Geometry: final body of the model. Coordinates: model frame, mm. A direction names the side the tool comes from. Give positions to 0.01 mm unless a question says otherwise; leave off trailing zeros. Write each loop counter-clockwise with the first axis right and the second up, starting at its lowest first coordinate (ties: lowest second). Pieces come first, ordered by that corner, then holes. Notation, with made-up numbers: (56, 55.25) -> (76, 55.25) arc R26 ccw to (76, 75.25) -> close; hole circle Ø8 at (9, 22). An arc over 180 degrees is marked (long way). Use CSV: the item, a comma, the result in double quotes. Start each with the question number.
1) Contact query for flat-ended pins moving along their axis: P1, Ø7, axis at y = -5.5, z = 0.5, coming from the +X side; P2, Ø7.5, axis at x = 13, y = -8, coming from the -Z side; P3, Ø5.5, axis at x = -7.5, z = -14, coming from the -Y side. Output: stop coordinate, or through.
2) Material intervals for line 1 (Z direction, x = 24.5, y = -3.75); line 2 (Y direction, x = -10.5, z = -23.5); line 3 (X direction, y = -6.5, z = -16.5), sorted ascending. Write a range as [from, to].
3) Set-up query: faces 5 (the face through (16, -5, -6.35)), 6 (the face through (29.21, 1, -1)), 7 (the face through (-8, 0, -14)). Return all of +Z, -Z, +X, -X, +Y, -Y with unobstructed straight access to the full face (end or side cutting, diameter ignored); none if empty.
4) Draft query along Z for faces 1 (the face through (17, -6, -3.81)), 2 (the face through (-15.315, 1.164, -24.887)), 3 (the face through (-11.635, -12.519, -12.151)), 4 (the face through (-13.49, -12.51, -11.03)). Return one class per face: pulls with the +Z half, pulls with the -Z half, needs draft (parallel to the pull), parting line crosses it, or undercut.
5) Section B-B (x = 24.5). Output: boundary loops of the cut face in (y, z) (3 decimals).
```python
from build123d import *

# Parameters (mm, degrees)
F1_DEPTH = 12.7
F3_DEPTH = 3.81
F4_R     = 0.635


with BuildPart() as f1:
    # F0 (on Front) → F1 (new body)
    with BuildSketch(Plane.XZ):
        with BuildLine():
            Line((4.445, 3.81), (29.21, 3.81))
            Line((29.21, 3.81), (29.21, 6.35))
            Line((29.21, 6.35), (3.6661742094, 6.35))
            ThreePointArc((3.6661742094, 6.35), (-2.6838257906, 4.6485226281), (-7.3323484187, 0))
            Line((-7.3323484187, 0), (-20.104261314, -22.1216020445))
            Line((-20.104261314, -22.1216020445), (-17.9045567884, -23.3916020445))
            Line((-17.9045567884, -23.3916020445), (-5.5220567884, -1.9444829198))
            ThreePointArc((-5.5220567884, -1.9444829198), (-5.1364807507, -1.6486200201), (-4.654630657, -1.7120567884))
            Line((-4.654630657, -1.7120567884), (0.844630657, -4.8870567884))
            ThreePointArc((0.844630657, -4.8870567884), (1.1404935567, -5.2726328262), (1.0770567884, -5.7544829198))
            Line((1.0770567884, -5.7544829198), (-11.3054432116, -27.2016020445))
            Line((-11.3054432116, -27.2016020445), (-9.105738686, -28.4716020445))
            Line((-9.105738686, -28.4716020445), (3.6661742094, -6.35))
            Line((3.6661742094, -6.35), (29.21, -6.35))
            Line((29.21, -6.35), (29.21, -3.81))
            Line((29.21, -3.81), (4.445, -3.81))
            ThreePointArc((4.445, -3.81), (3.9959871939, -3.6240128061), (3.81, -3.175))
            Line((3.81, -3.175), (3.81, 3.175))
            ThreePointArc((3.81, 3.175), (3.9959871939, 3.6240128061), (4.445, 3.81))
        make_face()
    extrude(amount=F1_DEPTH)

    # F2 (on face) → F3 (join)
    with BuildSketch(Plane(origin=(0, 0, 0), x_dir=(-1, 0, 0), z_dir=(0, 1, 0))):
        with BuildLine():
            Line((-3.6661742094, 6.35), (-29.21, 6.35))
            Line((-29.21, 6.35), (-29.21, -6.35))
            Line((-29.21, -6.35), (-3.6661742094, -6.35))
            Line((-3.6661742094, -6.35), (9.105738686, -28.4716020445))
            Line((9.105738686, -28.4716020445), (11.3054432116, -27.2016020445))
            Line((11.3054432116, -27.2016020445), (20.104261314, -22.1216020445))
            Line((20.104261314, -22.1216020445), (7.3323484187, 0))
            ThreePointArc((7.3323484187, 0), (2.6838257906, 4.6485226281), (-3.6661742094, 6.35))
        make_face()
    extrude(amount=F3_DEPTH)

    # F4
    f4_edges = [f1.edges().sort_by_distance(p)[0] for p in [
        (-2.719782, -12.7, -17.410801),
        (16.438087, -12.7, -6.35),
        (29.21, -12.7, -5.08),
        (16.8275, -12.7, -3.81),
        (3.995987, -12.7, -3.624013),
        (3.81, -12.7, 0),
        (3.995987, -12.7, 3.624013),
        (16.8275, -12.7, 3.81),
        (29.21, -12.7, 5.08),
        (16.438087, -12.7, 6.35),
        (-2.683826, -12.7, 4.648523),
        (-13.718305, -12.7, -11.060801),
        (-19.004409, -12.7, -22.756602),
        (-11.713307, -12.7, -12.668042),
        (-5.136481, -12.7, -1.64862),
        (-1.905, -12.7, -3.299557),
        (1.140494, -12.7, -5.272633),
        (-5.114193, -12.7, -16.478042),
        (-10.205591, -12.7, -27.836602),
        (29.21, -6.35, -3.81),
        (29.21, 0, 0),
        (29.21, -6.35, 3.81),
        (29.21, -4.445, 6.35),
        (29.21, 3.81, 0),
        (29.21, -4.445, -6.35),
        (-11.305443, -6.35, -27.201602),
        (-9.105739, -4.445, -28.471602),
        (-14.605, 3.81, -25.296602),
        (-20.104261, -4.445, -22.121602),
        (-17.904557, -6.35, -23.391602),
        (-14.605, 0, -25.296602),
        (16.438087, 3.81, 6.35),
        (16.438087, 3.81, -6.35),
        (-2.719782, 3.81, -17.410801),
        (-13.718305, 3.81, -11.060801),
        (-2.683826, 3.81, 4.648523),
        (3.666174, -4.445, -6.35),
    ]]
    fillet(f4_edges, radius=F4_R)


solid = f1.part
```
Answers follow:
1,P1,"stops at x = 29.03"
1,P2,"stops at z = -6.35"
1,P3,"stops at y = 0"
2,line 1,"z = [-6.35, -3.81], [3.81, 6.35]"
2,line 2,"y = [0, 3.81]"
2,line 3,"x = [-16.86, -13.93], [-5.13, -2.19]"
3,face 5,"-Z, +X, +Y, -Y"
3,face 6,"+Z, -Z, +X, +Y, -Y"
3,face 7,"-Y"
4,face 1,"undercut"
4,face 2,"pulls with the -Z half"
4,face 3,"undercut"
4,face 4,"pulls with the +Z half"
5,outline,"(-12.7, -5.715) arc R0.635 ccw to (-12.065, -6.35) -> (3.175, -6.35) arc R0.635 ccw to (3.81, -5.715) -> (3.81, 5.715) arc R0.635 ccw to (3.175, 6.35) -> (-12.065, 6.35) arc R0.635 ccw to (-12.7, 5.715) -> (-12.7, 4.445) arc R0.635 ccw to (-12.065, 3.81) -> (0, 3.81) -> (0, -3.81) -> (-12.065, -3.81) arc R0.635 ccw to (-12.7, -4.445) -> close"
